Verification items for the finished model (mm, model axes). A direction names the side the tool comes from. Coordinates: 2 decimals unless noted, no trailing zeros. Order: outer loops, then holes, each group sorted by start corner. A loop starts at its lowest first (then second) coordinate and runs counter-clockwise, first axis right, second up. Notation, with made-up numbers: M 56,2 L 67,2 A27 ccw 67,41 Z; hole C 56.25,45.25 d8. An arc over 180 degrees is marked long. Answer as a JSON object with one key per item and string values. Group by question number.
(1) Cross-section at C-C (x = -22). Enter the section's corners in (y, z).
(2) Access from +Z, -Z, +X, -X, +Y, -Y to the whole of each face (thin tool, end or side, straight path). Record for faces 4 (the face through (-16, 5.922, -5)), 5 (the face through (-16, 0, 1)), 6 (the face through (-16, 5.922, 7)), 7 (the face through (-17, 0, -10)).
(3) Cross-section at D-D (z = 4.5). Count the separate pieces of the cut face and the enclosed holes in it, plus the area to 3 significant figures.
(4) Mould release check, pull along Z, two halves, no side actions. Record for faces 1 (the face through (-16, 0, -1)), 2 (the face through (14.986, -0.126, -0.646)), 3 (the face through (-17, 0, 10)): released by +Z, released by -Z, zero draft, split by the parting line, or undercut.
(5) Gauge pin test, flat ends, axial feed: pin 1 Ø2.5 at (x, z) = (-16, -5) entering from +Y; pin 2 Ø6 at (x, y) = (-18, -1.5) entering from +Z; pin 3 Ø8 at (x, y) = (-22, 2.5) entering from -Z; pin 4 Ø3 at (x, y) = (-20, 0) entering from +Z. Record the tip position at first contact, or that the pin passes through.
(6) Cross-section at B-B (y = 0). Enter the section's corners in (x, z).
(7) Material ranges on line 1 (Y direction, x = -20, z = 4.5); line 2 (Z direction, x = -12, y = 0); line 3 (X direction, y = 1.75, z = -12), recorded low to high.
(8) Cross-section at A-A (x = 0). Enter the section's corners in (y, z), plus the area to 3 significant figures.
from build123d import *

# Parameters (mm, degrees)
F0_R          = 15
F0_R_2        = 10
F1_DEPTH      = 10
F1_DEPTH_BACK = 10
F2_R          = 2.5
F3_DEPTH      = 10
F3_DEPTH_BACK = 10
F4_W          = 50
F4_H          = 2
F5_DEPTH      = 25
F5_DEPTH_BACK = 25
F6_R          = 1


with BuildPart() as f1:
    # F0 (on Front) → F1 (new body, two sides)
    with BuildSketch(Plane.XZ) as f1_sk:
        Circle(F0_R)
        Circle(F0_R_2, mode=Mode.SUBTRACT)
    extrude(amount=F1_DEPTH)
    extrude(f1_sk.sketch, amount=-F1_DEPTH_BACK)

    # F2 (on Top) → F3 (join, two sides)
    with BuildSketch(Plane.XY) as f3_sk:
        with BuildLine():
            Line((-10.9971821198, 5.9223911099), (-19.0380834019, 5.9223911099))
            ThreePointArc((-19.0380834019, 5.9223911099), (-25.9784366079, 0.5082280244), (-20.0515892658, -5.9997782082))
            Line((-20.0515892658, -5.9997782082), (-11, -6.0776085593))
            Line((-11, -6.0776085593), (-10.9971821198, 5.9223911099))
        make_face()
        with Locations((-20, 0)):
            Circle(F2_R, mode=Mode.SUBTRACT)
    extrude(amount=F3_DEPTH)
    extrude(f3_sk.sketch, amount=-F3_DEPTH_BACK)

    # F4 (on Front) → F5 (cut, two sides)
    with BuildSketch(Plane.XZ) as f5_sk:
        with Locations((-31.5975938924, 0)):
            Rectangle(F4_W, F4_H)
    extrude(amount=-F5_DEPTH, mode=Mode.SUBTRACT)
    extrude(f5_sk.sketch, amount=F5_DEPTH_BACK, mode=Mode.SUBTRACT)

    # F6
    f6_edges = [f1.edges().sort_by_distance(p)[0] for p in [
        (15, -10, 0),
        (15, 10, 0),
    ]]
    fillet(f6_edges, radius=F6_R)


solid = f1.part
Taken from the geometry:
{
 "1": {"outline": "M -5.66,-10 L -1.5,-10 L -1.5,-1 L -5.66,-1 Z; M -5.66,1 L -1.5,1 L -1.5,10 L -5.66,10 Z; M 1.5,-10 L 5.66,-10 L 5.66,-1 L 1.5,-1 Z; M 1.5,1 L 5.66,1 L 5.66,10 L 1.5,10 Z"},
 "2": {"face 4": "-Z, +Y", "face 5": "-X, +Y, -Y", "face 6": "+Z, +Y", "face 7": "-Z, -X, +Y, -Y"},
 "3": {"separate pieces": "2", "enclosed holes": "1", "area": "319 mm²"},
 "4": {"face 1": "undercut", "face 2": "split by the parting line", "face 3": "released by +Z"},
 "5": {"pin 1": "stops at y = 5.92", "pin 2": "stops at z = 10", "pin 3": "stops at z = -10", "pin 4": "passes through"},
 "6": {"outline": "M -26,-10 L -22.5,-10 L -22.5,-1 L -26,-1 Z; M -26,1 L -22.5,1 L -22.5,10 L -26,10 Z; M -17.5,-10 L -11.18,-10 A15 ccw long -11.18,10 L -17.5,10 L -17.5,1 L -9.95,1 A10 cw long -9.95,-1 L -17.5,-1 Z"},
 "7": {"line 1": "y = -6 to -2.5, 2.5 to 6", "line 2": "z = -10 to -1, 1 to 10", "line 3": "x = -9 to 9"},
 "8": {"outline": "M -10,-14 A1 ccw -9,-15 L 9,-15 A1 ccw 10,-14 L 10,-10 L -10,-10 Z; M -10,10 L 10,10 L 10,14 A1 ccw 9,15 L -9,15 A1 ccw -10,14 Z", "area": "199 mm²"}
}
